from build123d import *

# Parameters (mm, degrees)
SKETCH1_R                = 19.7
SKETCH1_R_2              = 11.7
BOSS_EXTRUDE1_DEPTH      = 0.75
M2_CLEARANCE_HOLE1_D     = 2.4
M2_CLEARANCE_HOLE1_DEPTH = 1.5


with BuildPart() as part:
    # Sketch1 → Boss-Extrude1 (new body, symmetric)
    with BuildSketch(Plane.XY):
        Circle(SKETCH1_R)
        Circle(SKETCH1_R_2, mode=Mode.SUBTRACT)
    extrude(amount=BOSS_EXTRUDE1_DEPTH, both=True)

    # M2 Clearance Hole1
    with Locations(Plane.XY.offset(0.75)):
        with Locations((-12.990381057, 7.5), (0, 15), (12.990381057, 7.5), (12.990381057, -7.5), (0, -15), (-12.990381057, -7.5)):
            Hole(M2_CLEARANCE_HOLE1_D / 2, depth=M2_CLEARANCE_HOLE1_DEPTH)


solid = part.part
Part model, mm, in its own coordinate system. Give positions to 0.01 mm unless a question says otherwise; leave off trailing zeros. Loops run counter-clockwise (first coordinate to the right, second up) from the corner with the lowest first, then second, coordinate; pieces in that order, holes last.
(1) Band-saw the part on D-D (y = 7.5). Write the cut outline in (x, z), and give its area (3 significant figures).
Return value:
outline: (-18.22, -0.75) - (-14.19, -0.75) - (-14.19, 0.75) - (-18.22, 0.75) - close; (-11.79, -0.75) - (-8.98, -0.75) - (-8.98, 0.75) - (-11.79, 0.75) - close; (8.98, -0.75) - (11.79, -0.75) - (11.79, 0.75) - (8.98, 0.75) - close; (14.19, -0.75) - (18.22, -0.75) - (18.22, 0.75) - (14.19, 0.75) - close
area: 20.5 mm2
(2) Band-saw the part on B-B (z = -0.3). Write the cut outline in (x, y), and give its area (3 significant figures).
Return value:
outline: circle Ø39.4 at (0, 0); hole circle Ø2.4 at (-12.99, -7.5); hole circle Ø2.4 at (-12.99, 7.5); hole circle Ø23.4 at (0, 0); hole circle Ø2.4 at (0, -15); hole circle Ø2.4 at (0, 15); hole circle Ø2.4 at (12.99, -7.5); hole circle Ø2.4 at (12.99, 7.5)
area: 762 mm2
(3) Pull direction X, two halves, no side cores. Call faces 1 (the cylindrical face through (0.26, 13.83, -0.01)), 2 (the cylindrical face through (-2.54, -11.42, -0.01)), 3 (the flat face through (8.5, -8.5, 0.75)), 4 (the cylindrical face through (-15.63, -11.99, 0.01)): pulls with the +X half, pulls with the -X half, needs draft (parallel to the pull), parting line crosses it, or undercut.
Return value:
face 1: undercut
face 2: undercut
face 3: needs draft
face 4: parting line crosses it
(4) Drill centre lines: line 1 along Y through (x, z) = (0, 0.15); line 2 along X through (y, z) = (-0.5, 0.2); line 3 along Y through (x, z) = (-7, -0.5). Where is each one in solid material? Low to high.
Return value:
line 1: y = -19.7 to -16.2, -13.8 to -11.7, 11.7 to 13.8, 16.2 to 19.7
line 2: x = -19.69 to -11.69, 11.69 to 19.69
line 3: y = -18.41 to -9.37, 9.37 to 18.41
(5) Band-saw the part on C-C (x = 0). Write the cut outline in (y, z).
Return value:
outline: (-19.7, -0.75) - (-16.2, -0.75) - (-16.2, 0.75) - (-19.7, 0.75) - close; (-13.8, -0.75) - (-11.7, -0.75) - (-11.7, 0.75) - (-13.8, 0.75) - close; (11.7, -0.75) - (13.8, -0.75) - (13.8, 0.75) - (11.7, 0.75) - close; (16.2, -0.75) - (19.7, -0.75) - (19.7, 0.75) - (16.2, 0.75) - close
(6) Band-saw the part on A-A (y = 0). Write the cut outline in (x, z).
Return value:
outline: (-19.7, -0.75) - (-11.7, -0.75) - (-11.7, 0.75) - (-19.7, 0.75) - close; (11.7, -0.75) - (19.7, -0.75) - (19.7, 0.75) - (11.7, 0.75) - close
